Part model, mm, in its own coordinate system. A direction names the side the tool comes from. Coordinates: 2 decimals unless noted, no trailing zeros.
from build123d import *

# Parameters (mm, degrees)
BOSS_EXTRUDE1_DEPTH      = 0.5
BOSS_EXTRUDE1_DEPTH_BACK = 0.5
BOSS_EXTRUDE2_START      = -0.5
SKETCH2_R                = 1.75
SKETCH2_R_2              = 1
BOSS_EXTRUDE2_DEPTH      = 1
FILLET1_R                = 2.5
CUT_EXTRUDE1_DEPTH       = 12.332242011
CUT_EXTRUDE1_DEPTH_BACK  = 12.332242011
SKETCH2_2_R              = 1
FILLET4_R                = 0.25


with BuildPart() as part:
    # Sketch1 → Boss-Extrude1 (new, two sides: drawn at the far end of the back side and taken through both)
    with BuildSketch(Plane.XY.offset(-BOSS_EXTRUDE1_DEPTH_BACK)):
        with BuildLine():
            ThreePointArc((8, 0), (6.782329983, 4.242640687), (3.5, 7.193747285))
            Line((3.5, 7.193747285), (2.40625, 4.945701258))
            ThreePointArc((2.40625, 4.945701258), (4.662851863, 2.916815472), (5.5, 0))
            ThreePointArc((5.5, 0), (-2.916815472, -4.662851863), (-2.40625, 4.945701258))
            Line((-2.40625, 4.945701258), (-3.5, 7.193747285))
            ThreePointArc((-3.5, 7.193747285), (-4.242640687, -6.782329983), (8, 0))
        make_face()
    extrude(amount=BOSS_EXTRUDE1_DEPTH + BOSS_EXTRUDE1_DEPTH_BACK)

    # Sketch2 → Boss-Extrude2 (add)
    # profile 1 of 2: a face of its own
    with BuildSketch(Plane.XY.offset(BOSS_EXTRUDE2_START)):
        with Locations((-4.980451069, 6.260599584)):
            Circle(SKETCH2_R)
        with Locations((-4.980451069, 6.260599584)):
            Circle(SKETCH2_R_2, mode=Mode.SUBTRACT)
    # profile 2 of 2: a face of its own
    with BuildSketch(Plane.XY.offset(BOSS_EXTRUDE2_START)):
        with Locations((4.980451069, 6.260599584)):
            Circle(SKETCH2_R)
        with Locations((4.980451069, 6.260599584)):
            Circle(SKETCH2_R_2, mode=Mode.SUBTRACT)
    extrude(amount=BOSS_EXTRUDE2_DEPTH)

    # Fillet1
    fillet1_edges = [part.edges().sort_by_distance(p)[0] for p in [
        (-6.222579772, 5.02787241, 0),
        (6.222579772, 5.02787241, 0),
    ]]
    fillet(fillet1_edges, radius=FILLET1_R)

    # Sketch2<2> → Cut-Extrude1 (cut, two sides: drawn at the far end of the back side and taken through both)
    with BuildSketch(Plane.XY.offset(-CUT_EXTRUDE1_DEPTH_BACK)):
        with Locations((-4.980451069, 6.260599584)):
            Circle(SKETCH2_2_R)
        with Locations((4.980451069, 6.260599584)):
            Circle(SKETCH2_2_R)
    extrude(amount=CUT_EXTRUDE1_DEPTH + CUT_EXTRUDE1_DEPTH_BACK, mode=Mode.SUBTRACT)

    # Fillet4
    fillet4_edges = [part.edges().sort_by_distance(p)[0] for p in [
        (0, -5.5, 0.5),
        (0, -5.5, -0.5),
        (2.40625, 4.945701258, 0),
        (-2.40625, 4.945701258, 0),
    ]]
    fillet(fillet4_edges, radius=FILLET4_R)


solid = part.part
Q1. Wall check: line 1 along X through (y, z) = (6.5, 0.2); line 2 along Y through (x, z) = (4.75, -0.2); line 3 along Y through (x, z) = (-4.5, -0.05). Give the ranges that are in metal, low to high.
Results list:
line 1: x = -6.71 to -5.95, -4.01 to -3.16, 3.16 to 4.01, 5.95 to 6.71
line 2: y = -6.44 to -2.77, 2.77 to 5.29, 7.23 to 8
line 3: y = -6.61 to -3.16, 3.16 to 5.38, 7.14 to 7.94
Q2. Pin check, flat tip, straight feed: pin 1 Ø5 at (x, y) = (-1.5, -2) entering from +Z. Stop position of the tip, or through.
Results list:
pin 1: passes through
Q3. Mould opens along X. For faces 1 (the face through (-4.027, 6.561, -0.007)), 2 (the face through (0, -6, 0.5)) say: pulls with the +X half, pulls with the -X half, needs draft (parallel to the pull), parting line crosses it, or undercut.
Results list:
face 1: undercut
face 2: needs draft
Q4. Which spindle directions (+Z, -Z, +X, -X, +Y, -Y) get a long thin tool onto all of the face, cutting with end or side? Do faces 3 (the face through (0, -6, -0.5)), 4 (the face through (2.93, 6.02, -0.01)). Say none if no direction does.
Results list:
face 3: -Z, +X, -X, +Y, -Y
face 4: +Z, -Z, +Y
